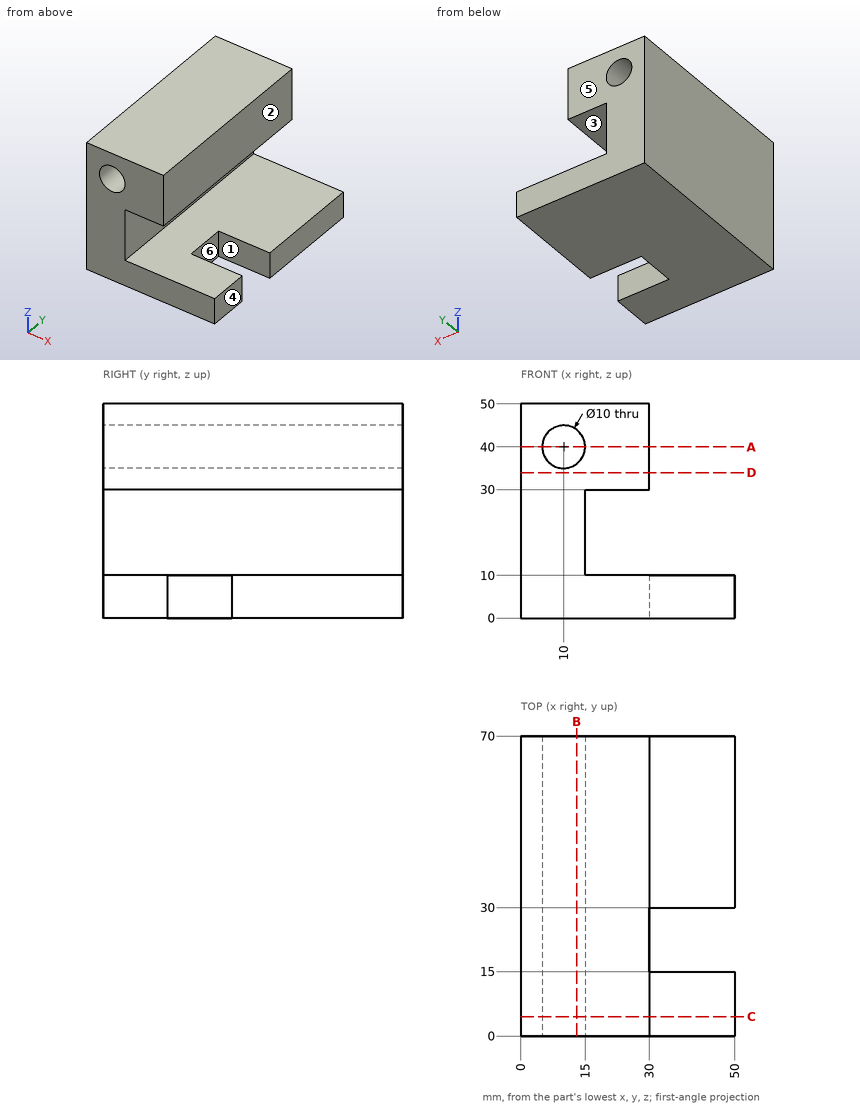
Study the drawing (mm; zero at the part's minimum x, y, z) and answer. A direction names the side the tool comes from. Give positions to 0.01 mm unless a question says otherwise; leave off trailing zeros. Write each loop counter-clockwise with the first axis right and the second up, starting at its lowest first coordinate (ties: lowest second). Pieces come first, ordered by that corner, then holes. Notation, with made-up numbers: M 57.25,49.25 L 83.25,49.25 A10 ccw 83.25,54.25 Z; hole C -8.5,79 d7. An arc over 180 degrees is marked long. Put each result on its own line as item: value. Start each with the question number.
1. The part is cut by section C-C, the plane y = 4.5. Give the vertices of the cut face in (x, z).
2. Each of these flat-tipped pins is pushed along its axis until it touches: pin 1 Ø16 at (y, z) = (44.5, 22.5) entering from +X; pin 2 Ø4 at (x, y) = (39.5, 17.5) entering from -Z. Where does it stop, or does it pass through?
3. Which of the six approach directions +Z, -Z, +X, -X, +Y, -Y give full straight-line access (tool end or side, diameter ignored) to the marked faces 1, 2 and 3?
4. The part is cut by section B-B, the plane x = 13. Give the vertices of the cut face in (y, z), and give its area (3 significant figures).
5. The part is cut by section D-D, the plane z = 34. Give the vertices of the cut face in (x, y), and give its area (3 significant figures).
6. For a pull along Y with two mould halves and no side action, classify the marked faces 4, 5 and 6 as released by +Y, released by -Y, zero draft, split by the parting line, or undercut.
7. Consider line 1 along Y through (x, z) = (43, 9); line 2 along Z through (x, y) = (15.5, 22.5); line 3 along Z through (x, y) = (10, 25). Determine where each line is inside the solid, lowest interval first.
8. The part is cut by section A-A, the plane z = 40. Give the vertices of the cut face in (x, y).
Final values:
1. outline: M 0,0 L 50,0 L 50,10 L 15,10 L 15,30 L 30,30 L 30,50 L 0,50 Z; hole C 10,40 d10
2. pin 1: stops at x = 30
2. pin 2: passes through
3. face 1: +Z, -Z, +X
3. face 2: +Z, +X, +Y, -Y
3. face 3: +X, +Y, -Y
4. outline: M 0,0 L 70,0 L 70,36 L 0,36 Z; M 0,44 L 70,44 L 70,50 L 0,50 Z
4. area: 2,940 mm²
5. outline: M 0,0 L 30,0 L 30,70 L 0,70 Z
5. area: 2,100 mm²
6. face 4: zero draft
6. face 5: released by +Y
6. face 6: undercut
7. line 1: y = 0 to 15, 30 to 70
7. line 2: z = 0 to 10, 30 to 50
7. line 3: z = 0 to 35, 45 to 50
8. outline: M 0,0 L 5,0 L 5,70 L 0,70 Z; M 15,0 L 30,0 L 30,70 L 15,70 Z
